from build123d import *

# Parameters (mm, degrees)
SKETCH1_W               = 203.2
SKETCH1_H               = 15.875
BOSS_EXTRUDE1_DEPTH     = 1.524
SKETCH5_R               = 3.175
BOSS_EXTRUDE5_DEPTH     = 15.875
CUT_EXTRUDE1_DEPTH      = 4.429
CUT_EXTRUDE1_DEPTH_BACK = 5.953


with BuildPart() as part:
    # Sketch1 → Boss-Extrude1 (new body)
    with BuildSketch(Plane(origin=(0, 0, 0), x_dir=(1, 0, 0), z_dir=(0, 1, 0))):
        Rectangle(SKETCH1_W, SKETCH1_H)
    extrude(amount=BOSS_EXTRUDE1_DEPTH)

    # Sketch5 → Boss-Extrude5 (add, through all)
    with BuildSketch(Plane.XY.offset(7.9375)):
        with BuildLine():
            ThreePointArc((-106.126651501, -2.065662651), (-104.000712573, -0.539318363), (-101.439759837, 0))
            Line((-101.439759837, 0), (-101.6, 0))
            Line((-101.6, 0), (-101.6, 1.524))
            Line((-101.6, 1.524), (-101.439759837, 1.524))
            ThreePointArc((-101.439759837, 1.524), (-104.000712573, 2.063318363), (-106.126651501, 3.589662651))
            ThreePointArc((-106.126651501, 3.589662651), (-113.411, 0.762), (-106.126651501, -2.065662651))
        make_face()
        with Locations((-109.22, 0.762)):
            Circle(SKETCH5_R, mode=Mode.SUBTRACT)
    boss_extrude5 = extrude(amount=-BOSS_EXTRUDE5_DEPTH)

    # Mirror1: Boss-Extrude5 across plane
    add(boss_extrude5.mirror(Plane(origin=(0, 0, 0), x_dir=(0, 0, 1), z_dir=(1, 0, 0))))

    # Sketch6 → Cut-Extrude1 (cut, two sides)
    with BuildSketch(Plane.XZ) as cut_extrude1_sk:
        Polygon((-113.411, -5.28621397), (-106.126651501, -7.9375), (-113.411, -7.9375), align=None)
        Polygon((-113.411, 7.9375), (-113.411, 5.28621397), (-106.126651501, 7.9375), align=None)
    extrude(amount=CUT_EXTRUDE1_DEPTH, mode=Mode.SUBTRACT)
    extrude(cut_extrude1_sk.sketch, amount=-CUT_EXTRUDE1_DEPTH_BACK, mode=Mode.SUBTRACT)


solid = part.part
Here's how the part is built. I have some questions about the finished solid (model axes, mm). A direction names the side the tool comes from. Coordinates: 2 decimals unless noted, no trailing zeros. Loops run counter-clockwise (first coordinate to the right, second up) from the corner with the lowest first, then second, coordinate; pieces in that order, holes last.
1. Imagine slicing it at B-B, the plane z = 1. Please give me the cut outline in (x, y) (3 decimals).
2. If we mould it in two halves opening along X, with no side actions, what happens to faces 1 (the flat face through (4, 1, -7.938)), 2 (the cylindrical face through (-104.034, -0.554, 0.111)), 3 (the flat face through (-112.214, 2.295, 5.722))? For each: pulls with the +X half, pulls with the -X half, needs draft (parallel to the pull), parting line crosses it, or undercut.
3. Imagine slicing it at A-A, the plane x = 109.22. Please give me the cut outline in (y, z).
4. For P1, Ø5, axis at x = 46, z = 2, coming from the -Y side; P2, Ø5, axis at x = -109.22, y = 0.762, coming from the -Z side; P3, Ø1, axis at y = 3.5, z = 5.5, coming from the -X side; P4, Ø8, axis at x = -43, z = -0.5, coming from the +Y side, each with a flat end and sliding along its axis, tell me the tip position at first contact or that it passes through.
5. Imagine slicing it at C-C, the plane x = -109.22. Please give me the cut outline in (y, z), and give its area (3 significant figures).
6. Imagine slicing it at D-D, the plane x = 5. Please give me the cut outline in (y, z), and give its area (3 significant figures).
7. I need wall thicknesses on L1, parallel to X at y = 0.5, z = -3.5; L2, parallel to X at y = 3.5, z = -3; L3, parallel to Y at x = 109.22, z = 0. Which ranges of each line are inside material? Lowest first, please.
8. For faces 4 (the cylindrical face through (-106.192, 1.716, 0.111)), 5 (the flat face through (-1, 0, 0)), 6 (the cylindrical face through (103.97, 2.05, 0.11)), which set-ups out of +Z, -Z, +X, -X, +Y, -Y let a thin tool reach every point of the face, with its end or its side?
Taken from the geometry:
1. outline: (-106.127, -2.066) arc R6.35 cw to (-101.44, 0) - (101.44, 0) arc R6.35 cw to (106.127, -2.066) arc R4.191 ccw (long way) to (106.127, 3.59) arc R6.35 cw to (101.44, 1.524) - (-101.44, 1.524) arc R6.35 cw to (-106.127, 3.59) arc R4.191 ccw (long way) to start; hole circle Ø6.35 at (-109.22, 0.762); hole circle Ø6.35 at (109.22, 0.762)
2. face 1: needs draft
2. face 2: undercut
2. face 3: pulls with the -X half
3. outline: (-3.43, -7.94) - (-2.41, -7.94) - (-2.41, 7.94) - (-3.43, 7.94) - close; (3.94, -7.94) - (4.95, -7.94) - (4.95, 7.94) - (3.94, 7.94) - close
4. P1: stops at y = 0
4. P2: passes through
4. P3: stops at x = -112.76
4. P4: stops at y = 1.52
5. outline: (-3.43, -6.81) - (-2.41, -6.81) - (-2.41, 6.81) - (-3.43, 6.81) - close; (3.94, -6.81) - (4.95, -6.81) - (4.95, 6.81) - (3.94, 6.81) - close
5. area: 27.7 mm2
6. outline: (0, -7.94) - (1.52, -7.94) - (1.52, 7.94) - (0, 7.94) - close
6. area: 24.2 mm2
7. L1: x = -113.4 to -112.38, -106.06 to 106.06, 112.38 to 113.4
7. L2: x = -112.39 to -110.83, -107.61 to -106.04, 106.04 to 107.61, 110.83 to 112.39
7. L3: y = -3.43 to -2.41, 3.94 to 4.95
8. face 4: +Z, -Z
8. face 5: +Z, -Z, -Y
8. face 6: +Z, -Z, +Y
